The figure shows three views and two pictorial views of one solid part (mm, origin at its lowest corner). Answer the questions. Give positions to 0.01 mm unless a question says otherwise; leave off trailing zeros. Write each loop counter-clockwise with the first axis right and the second up, starting at its lowest first coordinate (ties: lowest second). Pieces come first, ordered by that corner, then holes. Notation, with made-up numbers: (69, 58.25) - (81, 58.25) arc R25 cw to (81, 81.25) - close; hole circle Ø1 at (69, -4). An arc over 180 degrees is marked (long way). Use CSV: the item, a comma, the result in double quotes. Start each with the question number.
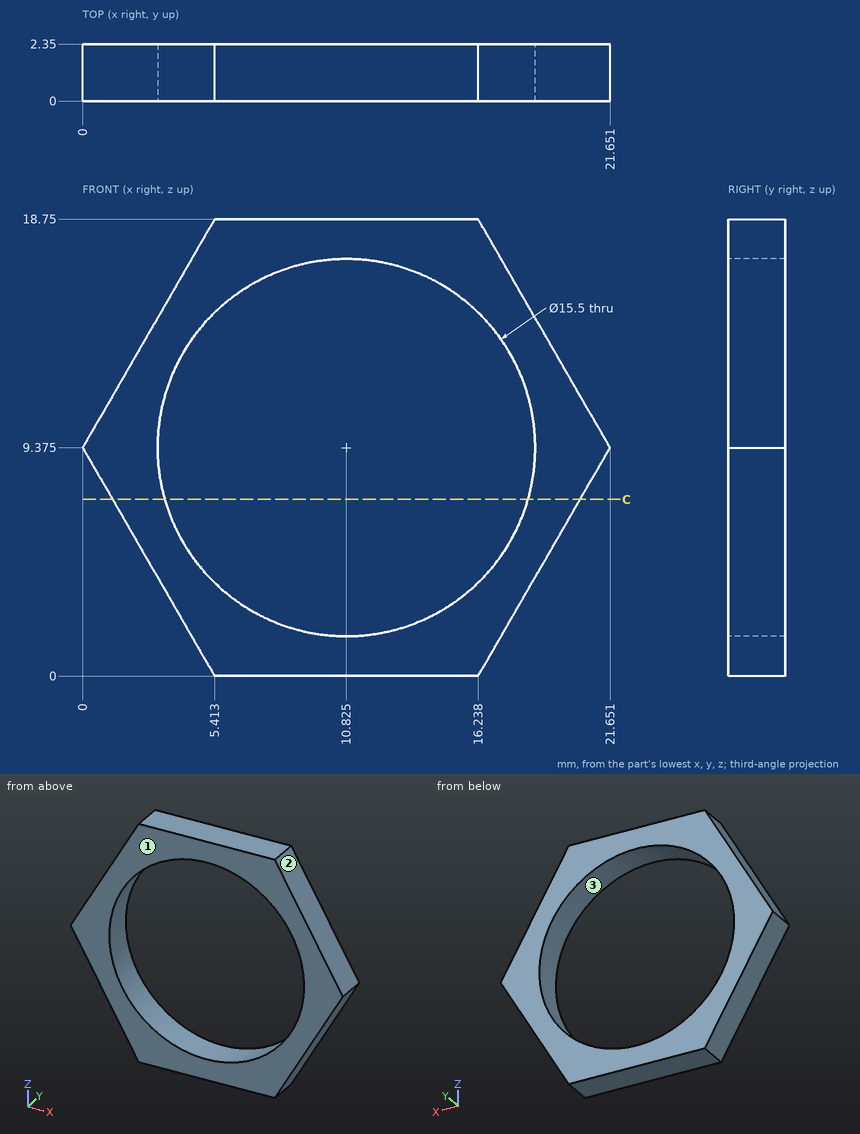
(1) The part is cut by section C-C on z = 7.25. Write down the section's boundary in (x, y), plus the area to 3 significant figures.
(2) Given P1, Ø1, axis at x = 18.5, y = 1, coming from the +Z side, flat-ended and moving along its own axis, determine where the tip first touches the part or whether it passes through.
(3) For a pull along X with two mould halves and no side action, classify the marked faces 1, 2 and 3 as pulls with the +X half, pulls with the -X half, needs draft (parallel to the pull), parting line crosses it, or undercut.
(4) Consider probe 1 along X at (y, z) = (1.4, 12.75); probe 2 along X at (y, z) = (0.3, 12.25); probe 3 along Z at (x, y) = (17.75, 1.3) (1 decimal). Determine where each line is inside the solid, lowest interval first.
Reported:
1,outline,"(1.23, 0) - (3.37, 0) - (3.37, 2.35) - (1.23, 2.35) - close; (18.28, 0) - (20.42, 0) - (20.42, 2.35) - (18.28, 2.35) - close"
1,area,"10.1 mm²"
2,P1,"z = 15.7"
3,face 1,"needs draft"
3,face 2,"pulls with the +X half"
3,face 3,"undercut"
4,probe 1,"1.95 to 3.85, 17.8 to 19.7"
4,probe 2,"1.66 to 3.63, 18.02 to 19.99"
4,probe 3,"2.6 to 5.9, 12.9 to 16.1"
